The listing builds one solid part. Answer for the finished solid, in the listing's coordinates (mm). Face numbers are marked on the shaded views. A direction names the side the tool comes from. Coordinates: 2 decimals unless noted, no trailing zeros. Write each loop counter-clockwise with the first axis right and the second up, starting at its lowest first coordinate (ties: lowest second). Pieces come first, ordered by that corner, then holes.
(1) The part is cut by section D-D on y = -4. Determine the outline of the cut face in (x, z), plus the area to 3 significant figures.
(2) The part is cut by section C-C on z = -179. Determine the outline of the cut face in (x, y), plus the area to 3 significant figures.
(3) For a pull along X with two mould halves and no side action, classify the marked faces 1, 2 and 3 as +X half, -X half, draft (parallel to the pull), parting line (faces both ways), or undercut.
(4) The part is cut by section B-B on x = 20. Determine the outline of the cut face in (y, z).
(5) The part is cut by section A-A on y = 15.5. Determine the outline of the cut face in (x, z).
(6) Given P1, Ø4, axis at x = -62.5, z = -226.5, coming from the +Y side; P2, Ø2.5, axis at x = 62.5, z = -115, coming from the +Y side; P3, Ø1.5, axis at x = 12.5, z = -57.5, coming from the +Y side; P4, Ø8, axis at x = 8, y = 19.5, coming from the +Z side, each flat-ended and moving along its own axis, determine where each tip first touches the part or whether it passes through.
(7) Which of the six approach directions +Z, -Z, +X, -X, +Y, -Y give full straight-line access (tool end or side, diameter ignored) to the marked faces 4 and 5?
(8) Straight lines are drawn through the part: line 1 (Z direction, x = -62.5, y = 33.5); line 2 (Z direction, x = 34, y = 28); line 3 (Y direction, x = -28, z = -3.25). For each, find the intervals that lie inside material, in ascending order.
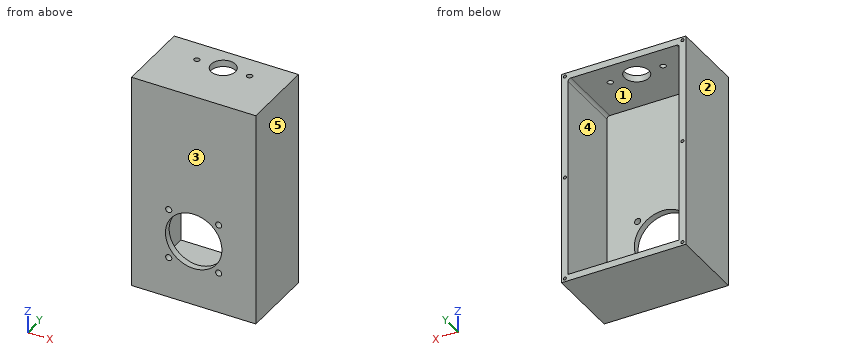
from build123d import *

# Parameters (mm, degrees)
SKETCH_1_W             = 132
SKETCH_1_H             = 80
EXTRUDE_1_DEPTH        = 230
SKETCH_2_W             = 118
SKETCH_2_H             = 216
CUT_EXTRUDE_1_DEPTH    = 73
SKETCH_3_R             = 13
SKETCH_3_R_2           = 3
CUT_EXTRUDE_2_DEPTH    = 10
SKETCH_4_R             = 3.25
SKETCH_4_R_2           = 30
CUT_EXTRUDE_3_DEPTH    = 10
FILLET_1_R             = 3
HOLE_WIZARD_M4_1_D     = 3.3
HOLE_WIZARD_M4_1_DEPTH = 10.1
HOLE_WIZARD_M4_1_TIP   = 0.991420021


with BuildPart() as part:
    # 草图1 → 凸台-拉伸1 (new body)
    with BuildSketch(Plane.XY):
        Rectangle(SKETCH_1_W, SKETCH_1_H)
    extrude(amount=-EXTRUDE_1_DEPTH)

    # 草图2 → 切除-拉伸1 (cut)
    with BuildSketch(Plane(origin=(0, 40, 0), x_dir=(1, 0, 0), z_dir=(0, 1, 0))):
        with Locations((0, 115)):
            Rectangle(SKETCH_2_W, SKETCH_2_H)
    extrude(amount=-CUT_EXTRUDE_1_DEPTH, mode=Mode.SUBTRACT)

    # 草图3 → 切除-拉伸2 (cut)
    with BuildSketch(Plane.XY):
        with Locations((0, 15.5)):
            Circle(SKETCH_3_R)
        with Locations((-28, 15.5)):
            Circle(SKETCH_3_R_2)
        with Locations((28, 15.5)):
            Circle(SKETCH_3_R_2)
    extrude(amount=-CUT_EXTRUDE_2_DEPTH, mode=Mode.SUBTRACT)

    # 草图4 → 切除-拉伸3 (cut)
    with BuildSketch(Plane(origin=(0, -33, 0), x_dir=(1, 0, 0), z_dir=(0, 1, 0))):
        with Locations((26.516504294, 186.516504294)):
            Circle(SKETCH_4_R)
        with Locations((26.516504294, 133.483495706)):
            Circle(SKETCH_4_R)
        with Locations((-26.516504294, 133.483495706)):
            Circle(SKETCH_4_R)
        with Locations((-26.516504294, 186.516504294)):
            Circle(SKETCH_4_R)
        with Locations((0, 160)):
            Circle(SKETCH_4_R_2)
    extrude(amount=-CUT_EXTRUDE_3_DEPTH, mode=Mode.SUBTRACT)

    # 圆角1
    fillet_1_edges = [part.edges().sort_by_distance(p)[0] for p in [
        (-59, 3.5, -7),
        (59, 3.5, -7),
    ]]
    fillet(fillet_1_edges, radius=FILLET_1_R)

    # M4 螺纹孔1
    with Locations(Plane(origin=(-62.5, 40, -226.5), x_dir=(0, 0, 1), z_dir=(0, 1, 0))):
        with Locations((0, 0), (111.5, 0), (111.5, 125), (0, 125), (223, 125), (223, 0)):
            Hole(HOLE_WIZARD_M4_1_D / 2, depth=HOLE_WIZARD_M4_1_DEPTH)
            with Locations((0, 0, -(HOLE_WIZARD_M4_1_DEPTH + HOLE_WIZARD_M4_1_TIP / 2))):  # 118° drill point
                Cone(0, HOLE_WIZARD_M4_1_D / 2, HOLE_WIZARD_M4_1_TIP, mode=Mode.SUBTRACT)


solid = part.part
Model answer:
1. outline: (-66, -230) - (66, -230) - (66, 0) - (-66, 0) - close; hole (-59, -223) - (59, -223) - (59, -10) arc R3 ccw to (56, -7) - (-56, -7) arc R3 ccw to (-59, -10) - close
1. area: 4,880 mm2
2. outline: (-66, -40) - (-23.22, -40) - (-23.22, -33) - (-59, -33) - (-59, 40) - (-66, 40) - close; (23.22, -40) - (66, -40) - (66, 40) - (59, 40) - (59, -33) - (23.22, -33) - close
2. area: 1,620 mm2
3. face 1: undercut
3. face 2: -X half
3. face 3: draft
4. outline: (-40, -230) - (40, -230) - (40, -223) - (-33, -223) - (-33, -182.36) - (-40, -182.36) - close; (-40, -137.64) - (-33, -137.64) - (-33, -7) - (40, -7) - (40, 0) - (-40, 0) - close
5. outline: (-66, -230) - (66, -230) - (66, 0) - (31, 0) - (31, -7) - (56, -7) arc R3 cw to (59, -10) - (59, -223) - (-59, -223) - (-59, -10) arc R3 cw to (-56, -7) - (-31, -7) - (-31, 0) - (-66, 0) - close; (-25, -7) - (-13, -7) - (-13, 0) - (-25, 0) - close; (13, -7) - (25, -7) - (25, 0) - (13, 0) - close
6. P1: stops at y = 40
6. P2: stops at y = 29.66
6. P3: stops at y = -33
6. P4: stops at z = -223
7. face 4: +Y
7. face 5: +Z, -Z, +X, +Y, -Y
8. line 1: z = -230 to -228.15, -224.85 to -116.65, -113.35 to -5.15, -1.85 to 0
8. line 2: z = -230 to -223, -7 to 0
8. line 3: y = -40 to 12.5, 18.5 to 40
